Build history of the part. All positions in model axes, mm. Face numbers are marked on the shaded views. A direction names the side the tool comes from. Give positions to 0.01 mm unless a question says otherwise; leave off trailing zeros. Order: outer loops, then holes, each group sorted by start corner. A loop starts at its lowest first (then second) coordinate and runs counter-clockwise, first axis right, second up. Notation, with made-up numbers: (-29, 67.5) -> (-14, 67.5) arc R19 cw to (-14, 101.5) -> close; hole circle Ø8 at (-22, -39). An arc over 180 degrees is marked (long way). One line per question, with ' | ' between items. Start each with the question number.
(1) Cut at C-C (x = -7.5). Give the cut face in (y, z), then the cut area to 4 significant figures.
(2) Drill centre lines: L1, parallel to X at y = -5.5, z = 17; L2, parallel to Z at x = -2.5, y = -4; L3, parallel to Y at x = 5, z = 6.5. Where is each one in solid material? Low to high. Write a range as from..to.
(3) Cut at B-B (y = -5). Give the cut face in (x, z).
(4) Cut at D-D (z = 16.5). Give the cut face in (x, y), then the cut area to 3 significant figures.
(5) Pull direction X, two halves, no side cores. Call the marked faces 1, 2 and 3: +X half, -X half, draft (parallel to the pull), parting line (faces both ways), or undercut.
(6) Which spindle directions (+Z, -Z, +X, -X, +Y, -Y) get a long thin tool onto all of the face, cutting with end or side? Do the marked faces 4, 5 and 6. Say none if no direction does.
(7) Pin check, flat tips, straight feed: pin 1 Ø1.5 at (x, y) = (-6.5, -2) entering from +Z; pin 2 Ø0.8 at (y, z) = (-2, 23.5) entering from -X; pin 3 Ø6 at (x, z) = (-1, 10) entering from -Y. Stop position of each tip, or through.
(8) Cut at A-A (x = 0). Give the cut face in (y, z), then the cut area to 4 significant figures.
from build123d import *

# Parameters (mm, degrees)
BOSS_EXTRUDE1_DEPTH      = 8.5
SKETCH2_W                = 17
SKETCH2_H                = 17
CUT_EXTRUDE1_DEPTH       = 6
CUT_EXTRUDE2_REACH       = 5
RESSALTO_EXTRUS_O1_DEPTH = 3
RESSALTO_EXTRUS_O2_DEPTH = 3
ESBO_O3_W                = 5
ESBO_O3_H                = 3
RESSALTO_EXTRUS_O3_DEPTH = 2.5


with BuildPart() as part:
    # Sketch1 → Boss-Extrude1 (new body, symmetric)
    with BuildSketch(Plane(origin=(0, 0, 0), x_dir=(0, 0, -1), z_dir=(1, 0, 0))):
        Polygon((0, 0), (-20, 0), (-20, -3), (-11.5, -11.5), (-3, -20), (0, -20), align=None)
    extrude(amount=BOSS_EXTRUDE1_DEPTH, both=True)

    # Sketch2 → Cut-Extrude1 (cut, symmetric)
    with BuildSketch(Plane(origin=(0, 0, 0), x_dir=(0, 0, -1), z_dir=(1, 0, 0))):
        with Locations((-11.5, -11.5)):
            Rectangle(SKETCH2_W, SKETCH2_H)
    extrude(amount=CUT_EXTRUDE1_DEPTH, both=True, mode=Mode.SUBTRACT)

    # Sketch3 → Cut-Extrude2 (cut, up to next)
    with BuildSketch(Plane.XY.offset(3), mode=Mode.PRIVATE) as cut_extrude2_sk1:
        with BuildLine():
            Line((-3, -9), (-3, -12))
            ThreePointArc((-3, -12), (0, -15), (3, -12))
            Line((3, -12), (3, -9))
            ThreePointArc((3, -9), (0, -6), (-3, -9))
        make_face()
    cut_extrude2_tool1 = extrude(cut_extrude2_sk1.sketch, amount=-CUT_EXTRUDE2_REACH, mode=Mode.PRIVATE) & part.part
    add(cut_extrude2_tool1.solids().sort_by_distance((0, -10.5, 3))[0], mode=Mode.SUBTRACT)

    # Esboço1 → Ressalto-extrusão1 (add)
    with BuildSketch(Plane.XY.offset(20)):
        Polygon((-8.5, 0), (-8.5, -3), (-6, -3), (6, -3), (8.5, -3), (8.5, 0), align=None)
    extrude(amount=RESSALTO_EXTRUS_O1_DEPTH)

    # Esboço2 → Ressalto-extrusão2 (add)
    with BuildSketch(Plane(origin=(0, 0, 0), x_dir=(1, 0, 0), z_dir=(0, 1, 0))):
        Polygon((-8.5, 0), (-12.433231648, -22.306465139), (-8.5, -23), align=None)
    ressalto_extrus_o2 = extrude(amount=-RESSALTO_EXTRUS_O2_DEPTH)

    # Esboço3 → Ressalto-extrusão3 (add)
    with BuildSketch(Plane.XY.offset(23)):
        with Locations((0, -1.5)):
            Rectangle(ESBO_O3_W, ESBO_O3_H)
    extrude(amount=RESSALTO_EXTRUS_O3_DEPTH)

    # Espelhar1: Ressalto-extrusão2 across plane
    add(ressalto_extrus_o2.mirror(Plane(origin=(0, 0, 0), x_dir=(0, 0, 1), z_dir=(1, 0, 0))))


solid = part.part
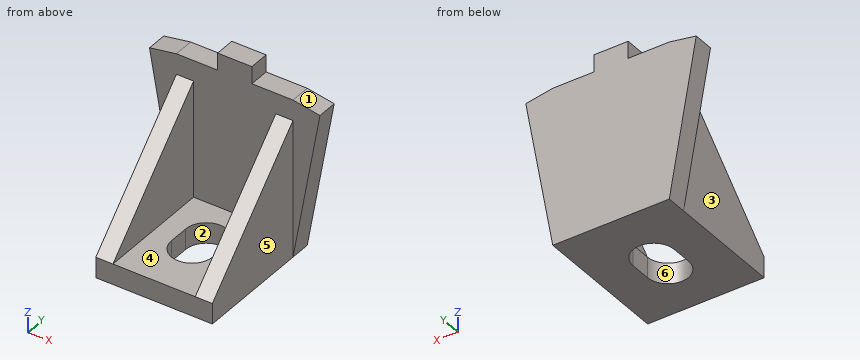
Result set:
1) outline: (-20, 0) -> (0, 0) -> (0, 23) -> (-3, 23) -> (-3, 20) -> (-20, 3) -> close | area: 264.5 mm2
2) L1: x = -8.5..-6, 6..8.5 | L2: z = 0..3 | L3: y = -3..0
3) outline: (-8.5, 0) -> (8.5, 0) -> (8.5, 18) -> (6, 18) -> (6, 3) -> (-6, 3) -> (-6, 18) -> (-8.5, 18) -> close
4) outline: (-11.41, -3) -> (-8.5, -3) -> (-8.5, -6.5) -> (-6, -6.5) -> (-6, -3) -> (6, -3) -> (6, -6.5) -> (8.5, -6.5) -> (8.5, -3) -> (11.41, -3) -> (11.41, 0) -> (-11.41, 0) -> close | area: 86.0 mm2
5) face 1: +X half | face 2: undercut | face 3: -X half
6) face 4: +Z, -Y | face 5: +Z, -Z, +X, -Y | face 6: +Z, -Z
7) pin 1: stops at z = 23 | pin 2: stops at x = -2.5 | pin 3: stops at y = -3
8) outline: (-20, 0) -> (-15, 0) -> (-15, 3) -> (-20, 3) -> close; (-6, 0) -> (0, 0) -> (0, 25.5) -> (-3, 25.5) -> (-3, 3) -> (-6, 3) -> close | area: 100.5 mm2
